from build123d import *

# Parameters (mm, degrees)
F2_SIZE = 1.4


# Not quite as in the source:
# - a fillet or chamfer that OpenCascade refuses, or shapes differently, is made with other operations: its cross-section is extruded or revolved along the edge and cut away or added


with BuildPart() as f1:
    # F0 (on Front) → F1 (revolve)
    with BuildSketch(Plane.XZ):
        with BuildLine():
            ThreePointArc((0, 0), (-3.8637033052, 2.9647238196), (-2, 7.4641016151))
            Line((-2, 7.4641016151), (-2, 10.4641016151))
            Line((-2, 10.4641016151), (-4, 10.4641016151))
            Line((-4, 10.4641016151), (-4, 8.472135955))
            ThreePointArc((-4, 8.472135955), (-5.6050341538, 1.8590674614), (0, -2))
            Line((0, -2), (0, 0))
        make_face()
    revolve(axis=Axis((0, 0, -1), (0, 0, -1)))

    # F2
    f2_edges = [f1.edges().sort_by_distance(p)[0] for p in [
        (2, 0, 10.464102),
    ]]
    chamfer(f2_edges, length=F2_SIZE)

    # F3: fillet of radius 8.5913249715 on 1 edges, made by hand

    # F3_s1 → F3_t2 (revolve)
    with BuildSketch(Plane.XZ):
        with BuildLine():
            ThreePointArc((-4, 10.4641016151), (-4.397901087, 8.7079815946), (-5.1530970812, 7.0733679363))
            ThreePointArc((-5.1530970812, 7.0733679363), (-4.6296797445, 7.8165515145), (-4, 8.472135955))
            Line((-4, 8.472135955), (-4, 10.4641016151))
        make_face()
    revolve(axis=Axis((0, 0, 8.472135955), (0, 0, -1)))


solid = f1.part
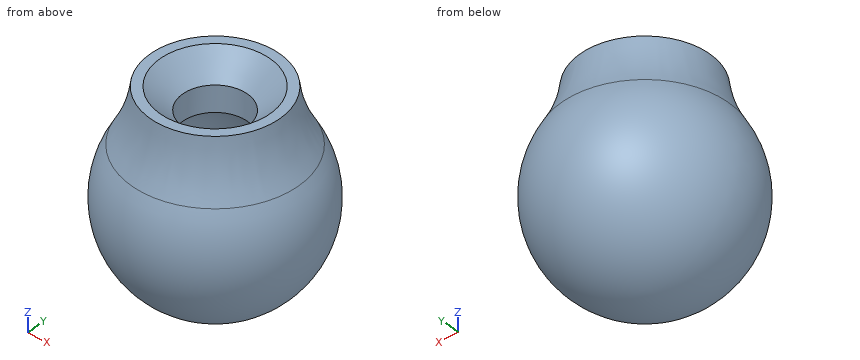
The model under review builds one solid part; all positions refer to its coordinate system, in mm. Give positions to 0.01 mm unless a question says otherwise; leave off trailing zeros. Order: outer loops, then holes, each group sorted by start corner. A loop starts at its lowest first (then second) coordinate and runs counter-clockwise, first axis right, second up. Notation, with made-up numbers: M 20,-27.5 L 55,-27.5 A12 cw 55,-6.5 Z; hole C 54,54.5 d11. An arc over 180 degrees is marked long. Use one line per item in the form item = value. Start each with the question number.
Item 1: Insertion check: pin 1 Ø3 at (x, y) = (-2.5, 1.5) entering from +Z; pin 2 Ø2 at (x, z) = (-0.5, 2) entering from -Y; pin 3 Ø3 at (y, z) = (-2.5, 7) entering from -X; pin 4 Ø1.5 at (x, z) = (-1.5, 6.5) entering from -Y. Each pin has a flat end and moves straight along its axis. Give the tip position at first contact, or say it passes through.
Item 2: We need section C-C on z = 8.5. Give the boundary of the cut face in (x, y), plus the area to 3 significant figures.
Item 3: We need section D-D on z = -0.25. Give the boundary of the cut face in (x, y).
Item 4: We need section A-A on y = 0. Give the boundary of the cut face in (x, z).
Item 5: To check wall thickness, follow line 1 along Y through (x, z) = (-4, 6); line 2 along X through (y, z) = (-1.5, 9.25); line 3 along Y through (x, z) = (1.75, 8.25). State the ranges of each line that lie inside material, in increasing order. Write a range as from..to.
Completed:
q1.pin_1 = 10.46
q1.pin_2 = -5.91
q1.pin_3 = -5.5
q1.pin_4 = -5.6
q2.outline = C 0,0 d8.94; hole C 0,0 d4
q2.area = 50.3 mm²
q3.outline = C 0,0 d8.47
q4.outline = M -5.15,7.07 A6 ccw long 5.15,7.07 A8.59 cw 4,10.46 L 3.4,10.46 L 2,9.06 L 2,7.46 A4 cw long -2,7.46 L -2,9.06 L -3.4,10.46 L -4,10.46 A8.59 cw Z
q5.line_1 = -4..4
q5.line_2 = -3.96..-1.59, 1.59..3.96
q5.line_3 = -4.22..-0.97, 0.97..4.22
